Verification items for the finished model (mm, model axes). Coordinates: 2 decimals unless noted, no trailing zeros. Loops run counter-clockwise (first coordinate to the right, second up) from the corner with the lowest first, then second, coordinate; pieces in that order, holes last. Notation, with made-up numbers: (-3.75, 66) - (0.25, 66) arc R18 ccw to (0.25, 101) - close; hole circle Ø11 at (70, 5). An arc over 180 degrees is marked (long way). Answer as CSV lines item,"result". Start each with the question number.
1. Gauge pin test, flat ends, axial feed: P1, Ø1.8, axis at x = -43.82, z = -19.88, coming from the +Y side; P2, Ø2.5, axis at x = -33.03, z = -19.88, coming from the +Y side; P3, Ø0.6, axis at x = -48, y = 0.5, coming from the +Z side. Record the tip position at first contact, or that the pin passes through.
2. Cross-section at C-C (y = 0.95). Enter the section's corners in (x, z), plus the area to 3 significant figures.
3. Cross-section at B-B (z = -14). Enter the section's corners in (x, y).
4. Cross-section at D-D (z = -19.5). Enter the section's corners in (x, y), plus the area to 3 significant figures.
5. Material ranges on line 1 (Z direction, x = -25.5, y = 1.05); line 2 (Z direction, x = -39, y = 0.2); line 3 (X direction, y = 0.7, z = -18.25), recorded low to high. Write a range as [from, to].
6. Cross-section at A-A (x = -38.5). Enter the section's corners in (y, z), plus the area to 3 significant figures.
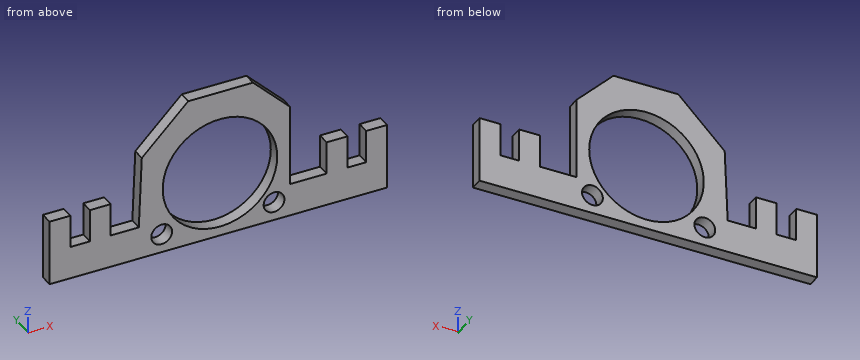
```python
from build123d import *

# Parameters (mm, degrees)
BOSS_EXTRUDE1_DEPTH = 1.2
CUT_EXTRUDE2_REACH  = 3.2
SKETCH3_R           = 1
SKETCH3_R_2         = 5.5


with BuildPart() as part:
    # Sketch1 → Boss-Extrude1 (new body)
    with BuildSketch(Plane(origin=(0, 0, 0), x_dir=(1, 0, 0), z_dir=(0, 1, 0))):
        Polygon((-54.589869364, 21.700331248), (-22.189869364, 21.700331248), (-22.189869364, 15.300331248), (-24.189869364, 15.300331248), (-24.189869364, 18.500331248), (-25.989869364, 18.500331248), (-25.989869364, 15.300331248), (-27.989869364, 15.300331248), (-27.989869364, 18.500331248), (-31.489869364, 18.500331248), (-31.489869364, 10.600331248), (-35.053687541, 7.036513071), (-41.273687541, 7.036513071), (-45.728460263, 11.491285792), (-46.013981929, 18.500331248), (-48.713981929, 18.500331248), (-48.713981929, 15.300331248), (-50.713981929, 15.300331248), (-50.713981929, 18.500331248), (-52.589869364, 18.500331248), (-52.589869364, 15.300331248), (-54.589869364, 15.300331248), align=None)
    extrude(amount=BOSS_EXTRUDE1_DEPTH)

    # Sketch3 → Cut-Extrude2 (cut, up to next)
    with BuildSketch(Plane(origin=(0, 1.2, 0), x_dir=(1, 0, 0), z_dir=(0, 1, 0)), mode=Mode.PRIVATE) as cut_extrude2_sk1:
        with Locations((-43.822096549, 19.883607228)):
            Circle(SKETCH3_R)
    cut_extrude2_tool1 = extrude(cut_extrude2_sk1.sketch, amount=-CUT_EXTRUDE2_REACH, mode=Mode.PRIVATE) & part.part
    add(cut_extrude2_tool1.solids().sort_by_distance((-43.822097, 1.2, -19.883607))[0], mode=Mode.SUBTRACT)
    # Sketch3 → Cut-Extrude2 (cut, up to next)
    with BuildSketch(Plane(origin=(0, 1.2, 0), x_dir=(1, 0, 0), z_dir=(0, 1, 0)), mode=Mode.PRIVATE) as cut_extrude2_sk2:
        with Locations((-33.032153908, 19.883607228)):
            Circle(SKETCH3_R)
    cut_extrude2_tool2 = extrude(cut_extrude2_sk2.sketch, amount=-CUT_EXTRUDE2_REACH, mode=Mode.PRIVATE) & part.part
    add(cut_extrude2_tool2.solids().sort_by_distance((-33.032154, 1.2, -19.883607))[0], mode=Mode.SUBTRACT)
    # Sketch3 → Cut-Extrude2 (cut, up to next)
    with BuildSketch(Plane(origin=(0, 1.2, 0), x_dir=(1, 0, 0), z_dir=(0, 1, 0)), mode=Mode.PRIVATE) as cut_extrude2_sk3:
        with Locations((-38.224033721, 15.300331248)):
            Circle(SKETCH3_R_2)
    cut_extrude2_tool3 = extrude(cut_extrude2_sk3.sketch, amount=-CUT_EXTRUDE2_REACH, mode=Mode.PRIVATE) & part.part
    add(cut_extrude2_tool3.solids().sort_by_distance((-38.224034, 1.2, -15.300331))[0], mode=Mode.SUBTRACT)


solid = part.part
```
Values follow:
1,P1,"passes through"
1,P2,"stops at y = 1.2"
1,P3,"stops at z = -18.5"
2,outline,"(-54.59, -21.7) - (-22.19, -21.7) - (-22.19, -15.3) - (-24.19, -15.3) - (-24.19, -18.5) - (-25.99, -18.5) - (-25.99, -15.3) - (-27.99, -15.3) - (-27.99, -18.5) - (-31.49, -18.5) - (-31.49, -10.6) - (-35.05, -7.04) - (-41.27, -7.04) - (-45.73, -11.49) - (-46.01, -18.5) - (-48.71, -18.5) - (-48.71, -15.3) - (-50.71, -15.3) - (-50.71, -18.5) - (-52.59, -18.5) - (-52.59, -15.3) - (-54.59, -15.3) - close; hole circle Ø2 at (-43.82, -19.88); hole circle Ø11 at (-38.22, -15.3); hole circle Ø2 at (-33.03, -19.88)"
2,area,"176 mm²"
3,outline,"(-45.83, 0) - (-43.57, 0) - (-43.57, 1.2) - (-45.83, 1.2) - close; (-32.88, 0) - (-31.49, 0) - (-31.49, 1.2) - (-32.88, 1.2) - close"
4,outline,"(-54.59, 0) - (-44.75, 0) - (-44.75, 1.2) - (-54.59, 1.2) - close; (-42.9, 0) - (-41.78, 0) - (-41.78, 1.2) - (-42.9, 1.2) - close; (-34.67, 0) - (-33.96, 0) - (-33.96, 1.2) - (-34.67, 1.2) - close; (-32.11, 0) - (-22.19, 0) - (-22.19, 1.2) - (-32.11, 1.2) - close"
4,area,"25.9 mm²"
5,line 1,"z = [-21.7, -18.5]"
5,line 2,"z = [-21.7, -20.75], [-9.86, -7.04]"
5,line 3,"x = [-54.59, -52.59], [-50.71, -48.71], [-46, -42.87], [-33.58, -31.49], [-27.99, -25.99], [-24.19, -22.19]"
6,outline,"(0, -21.7) - (1.2, -21.7) - (1.2, -20.79) - (0, -20.79) - close; (0, -9.81) - (1.2, -9.81) - (1.2, -7.04) - (0, -7.04) - close"
6,area,"4.41 mm²"
